```python
from build123d import *

# Parameters (mm, degrees)
BOSS_EXTRUDE1_DEPTH  = 3
SKETCH2_W            = 20
SKETCH2_H            = 56
BOSS_EXTRUDE2_DEPTH  = 0.5
SKETCH5_W            = 20
SKETCH5_H            = 56
BOSS_EXTRUDE3_DEPTH  = 0.5
SKETCH6_W            = 20
SKETCH6_H            = 56
BOSS_EXTRUDE4_DEPTH  = 0.5
SKETCH7_W            = 20
SKETCH7_H            = 56
BOSS_EXTRUDE5_DEPTH  = 0.5
BOSS_EXTRUDE18_DEPTH = 0.5
FILLET1_R            = 1


with BuildPart() as part:
    # Sketch1 → Boss-Extrude1 (new body)
    with BuildSketch(Plane.XY):
        with BuildLine():
            Line((0.088772672, 50.445513271), (0.088772672, 108.445513271))
            Line((0.088772672, 108.445513271), (20.088772672, 108.445513271))
            Line((20.088772672, 108.445513271), (20.088772672, 112.445513271))
            Line((20.088772672, 112.445513271), (40.088772672, 112.445513271))
            Line((40.088772672, 112.445513271), (40.088772672, 116.445513271))
            Line((40.088772672, 116.445513271), (60.088772672, 116.445513271))
            Line((60.088772672, 116.445513271), (60.088772672, 120.445513271))
            Line((60.088772672, 120.445513271), (80.088772672, 120.445513271))
            Line((80.088772672, 120.445513271), (80.088772672, 62.445513271))
            Line((80.088772672, 62.445513271), (95.696655206, 49.939754486))
            Line((95.696655206, 49.939754486), (79.719999866, 30))
            Line((79.719999866, 30), (79.719999866, 5))
            ThreePointArc((79.719999866, 5), (78.255533771, 1.464466094), (74.719999866, 0))
            Line((74.719999866, 0), (45.081340107, 0))
            Line((45.081340107, 0), (12.090244869, 0))
            ThreePointArc((12.090244869, 0), (10.402431062, 0.519821669), (9.299525382, 1.899143631))
            ThreePointArc((9.299525382, 1.899143631), (2.402932305, 25.737613543), (0.088772672, 50.445513271))
        make_face()
    extrude(amount=-BOSS_EXTRUDE1_DEPTH)

    # Sketch2 → Boss-Extrude2 (add)
    with BuildSketch(Plane.XY):
        with Locations((10.088772672, 80.445513271)):
            Rectangle(SKETCH2_W, SKETCH2_H)
    extrude(amount=BOSS_EXTRUDE2_DEPTH)

    # Sketch5 → Boss-Extrude3 (add)
    with BuildSketch(Plane.XY):
        with Locations((30.088772672, 84.445513271)):
            Rectangle(SKETCH5_W, SKETCH5_H)
    extrude(amount=BOSS_EXTRUDE3_DEPTH)

    # Sketch6 → Boss-Extrude4 (add)
    with BuildSketch(Plane.XY):
        with Locations((50.088772672, 88.445513271)):
            Rectangle(SKETCH6_W, SKETCH6_H)
    extrude(amount=BOSS_EXTRUDE4_DEPTH)

    # Sketch7 → Boss-Extrude5 (add)
    with BuildSketch(Plane.XY):
        with Locations((70.088772672, 92.445513271)):
            Rectangle(SKETCH7_W, SKETCH7_H)
    extrude(amount=BOSS_EXTRUDE5_DEPTH)

    # Sketch10 → Boss-Extrude18 (add)
    with BuildSketch(Plane.XY):
        Polygon((80.088772672, 62.445513271), (95.696655206, 49.939754486), (60.680530606, 6.23768339), (45.072648072, 18.743442176), align=None)
    extrude(amount=BOSS_EXTRUDE18_DEPTH)

    # Fillet1
    fillet1_edges = [part.edges().sort_by_distance(p)[0] for p in [
        (87.892713939, 56.192633878, -3),
        (80.088772672, 91.445513271, -3),
        (70.088772672, 120.445513271, -3),
        (60.088772672, 118.445513271, -3),
        (50.088772672, 116.445513271, -3),
        (40.088772672, 114.445513271, -3),
        (30.088772672, 112.445513271, -3),
        (20.088772672, 110.445513271, -3),
        (10.088772672, 108.445513271, -3),
        (0.088772672, 79.445513271, -3),
        (79.719999866, 17.5, -3),
        (2.402932305, 25.737613543, -3),
        (10.402431062, 0.519821669, -3),
        (43.405122367, 0, -3),
        (78.255533771, 1.464466094, -3),
        (87.708327536, 39.969877243, -3),
    ]]
    fillet(fillet1_edges, radius=FILLET1_R)


solid = part.part
```
The listing builds one solid part. Answer for the finished solid, in the listing's coordinates (mm). A direction names the side the tool comes from. Coordinates: 2 decimals unless noted, no trailing zeros. Write each loop counter-clockwise with the first axis right and the second up, starting at its lowest first coordinate (ties: lowest second). Pieces come first, ordered by that corner, then holes. Notation, with made-up numbers: (-27.5, -37.5) -> (-9.5, -37.5) arc R8 ccw to (-9.5, -24.5) -> close; hole circle Ø5 at (20, -4.75). An arc over 180 degrees is marked (long way). Write each question's results on one line, items separated by ' | '. Start each with the question number.
1) Flat-ended cylindrical pins translate along their axes: pin 1 Ø2 at (y, z) = (17.5, -1) entering from +X; pin 2 Ø0.6 at (y, z) = (58.5, 0.5) entering from +X; pin 3 Ø2 at (y, z) = (109.5, -1.5) entering from -X. Find the tip coordinate at first contact, or state that the pin passes through.
2) A cutting plane is placed at D-D (x = 53). Determine the outline of the cut face in (y, z).
3) Straight lines are drawn through the part: probe 1 along Y at (x, z) = (33, -0.25); probe 2 along Y at (x, z) = (49.5, -0.35); probe 3 along Y at (x, z) = (55.5, 0.15). For each, find the intervals that lie inside material, in ascending order.
4) A cutting plane is placed at A-A (x = 35.5). Determine the outline of the cut face in (y, z).
5) A cutting plane is placed at B-B (y = 92). Determine the outline of the cut face in (x, z), then the cut area to 3 significant figures.
6) For a pull along Y with two mould halves and no side action, classify faces 4 (the flat face through (41, 33, 0)), 5 (the flat face through (40.089, 114, -1)), 6 (the flat face through (70, 120.446, -1)) as +Y half, -Y half, draft (parallel to the pull), parting line (faces both ways), or undercut.
7) A tool of negligible diameter and unlimited length cuts with its end or side. For faces 1 (the flat face through (52.99, 12.4, 0.25)), 2 (the flat face through (62.336, 40.289, 0.246)), 3 (the flat face through (60.089, 118, -1)), from which of +Z, -Z, +X, -X, +Y, -Y can it reach the whole face along a straight path? Write none if from no direction.
8) A cutting plane is placed at C-C (z = -0.95). Determine the outline of the cut face in (x, y).
Values follow:
1) pin 1: x = 79.72 | pin 2: x = 85.39 | pin 3: x = 20.09
2) outline: (0, -2) arc R1 ccw to (1, -3) -> (115.45, -3) arc R1 ccw to (116.45, -2) -> (116.45, 0.5) -> (60.45, 0.5) -> (60.45, 0) -> (28.64, 0) -> (28.64, 0.5) -> (12.39, 0.5) -> (12.39, 0) -> (0, 0) -> close
3) probe 1: 0 to 112.45 | probe 2: 0 to 116.45 | probe 3: 10.39 to 31.76, 60.45 to 116.45
4) outline: (0, -2) arc R1 ccw to (1, -3) -> (111.45, -3) arc R1 ccw to (112.45, -2) -> (112.45, 0.5) -> (56.45, 0.5) -> (56.45, 0) -> (0, 0) -> close
5) outline: (0.09, -2) arc R1 ccw to (1.09, -3) -> (79.09, -3) arc R1 ccw to (80.09, -2) -> (80.09, 0.5) -> (0.09, 0.5) -> close | area: 280 mm²
6) face 4: undercut | face 5: draft | face 6: +Y half
7) face 1: +Z, -X, -Y | face 2: +Z | face 3: +Z, -Z, -X, +Y
8) outline: (0.09, 50.45) arc R132.04 ccw to (9.3, 1.9) arc R3 ccw to (12.09, 0) -> (74.72, 0) arc R5 ccw to (79.72, 5) -> (79.72, 30) -> (95.7, 49.94) -> (80.09, 62.45) -> (80.09, 120.45) -> (60.09, 120.45) -> (60.09, 116.45) -> (40.09, 116.45) -> (40.09, 112.45) -> (20.09, 112.45) -> (20.09, 108.45) -> (0.09, 108.45) -> close
